The listing builds one solid part. Answer for the finished solid, in the listing's coordinates (mm). Face numbers are marked on the shaded views. A direction names the side the tool comes from. Coordinates: 2 decimals unless noted, no trailing zeros. Write each loop counter-clockwise with the first axis right and the second up, starting at its lowest first coordinate (ties: lowest second). Pieces come first, ordered by that corner, then holes.
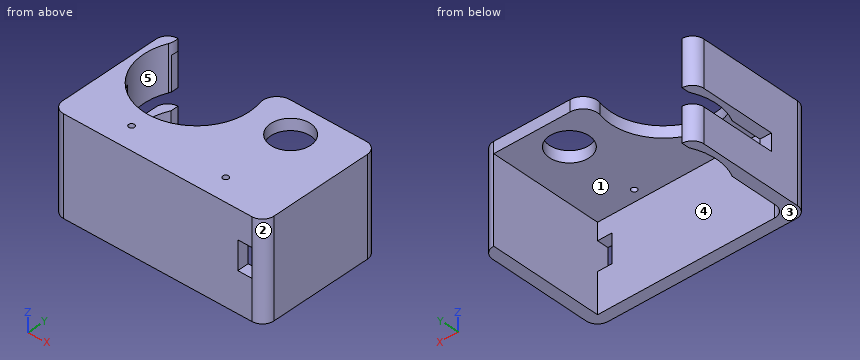
from build123d import *

# Parameters (mm, degrees)
ESQUISSE2_W             = 74
ESQUISSE2_H             = 44
BOSS_EXTRU_1_DEPTH      = 4
ESQUISSE4_R             = 7
ESQUISSE4_R_2           = 18.5
ESQUISSE4_R_3           = 1
ENL_V_MAT_EXTRU_1_DEPTH = 71.394310982
BOSS_EXTRU_2_START      = -4
BOSS_EXTRU_2_DEPTH      = 34
CONG_1_R                = 4
ESQUISSE7_W             = 6
ESQUISSE7_H             = 30
ENL_V_MAT_EXTRU_2_DEPTH = 10
CONG_2_START            = -13
CONG_2_DEPTH            = 18
ESQUISSE8_W             = 5
ESQUISSE8_H             = 10
ENL_V_MAT_EXTRU_3_DEPTH = 77.369560077


with BuildPart() as part:
    # Esquisse2 → Boss.-Extru.1 (new body)
    with BuildSketch(Plane.XY):
        with Locations((-20.726161369, 18.08801956)):
            Rectangle(ESQUISSE2_W, ESQUISSE2_H)
    extrude(amount=BOSS_EXTRU_1_DEPTH)

    # Esquisse4 → Enlèv. mat.-Extru.1 (cut, through all)
    with BuildSketch(Plane.XY.offset(4)):
        with Locations((-4.226161369, 29.08801956)):
            Circle(ESQUISSE4_R)
        with Locations((-37.226161369, 29.08801956)):
            Circle(ESQUISSE4_R_2)
        with Locations((-4.226161369, 4.08801956)):
            Circle(ESQUISSE4_R_3)
        with Locations((-37.226161369, 4.08801956)):
            Circle(ESQUISSE4_R_3)
    extrude(amount=-ENL_V_MAT_EXTRU_1_DEPTH, mode=Mode.SUBTRACT)

    # Boss.-Extru.2: read off the stored shape, not the designer's step
    # Boss.-Extru.2 outline → Boss.-Extru.2 (add)
    with BuildSketch(Plane(origin=(0, 0, 0), x_dir=(-1, 0, 0), z_dir=(0, 0, -1)).offset(BOSS_EXTRU_2_START)):
        with BuildLine():
            Line((-12.273838631, 40.08801956), (-16.273838631, 40.08801956))
            Line((-16.273838631, 40.08801956), (-16.273838631, -3.91198044))
            Line((-16.273838631, -3.91198044), (57.726161369, -3.91198044))
            Line((57.726161369, -3.91198044), (57.726161369, 40.08801956))
            Line((57.726161369, 40.08801956), (53.726161369, 40.08801956))
            Line((53.726161369, 40.08801956), (53.726161369, 37.454619825))
            ThreePointArc((53.726161369, 37.454619825), (55.726161369, 29.08801956), (53.726161369, 20.721419295))
            Line((53.726161369, 20.721419295), (53.726161369, 0.08801956))
            Line((53.726161369, 0.08801956), (-12.273838631, 0.08801956))
            Line((-12.273838631, 0.08801956), (-12.273838631, 40.08801956))
        make_face()
    extrude(amount=BOSS_EXTRU_2_DEPTH)

    # Congé1
    cong_1_edges = [part.edges().sort_by_distance(p)[0] for p in [
        (-53.726161369, 0.08801956, -15),
        (-57.726161369, 40.08801956, -15),
        (16.273838631, 40.08801956, -15),
        (16.273838631, -3.91198044, -15),
        (-57.726161369, -3.91198044, -15),
    ]]
    fillet(cong_1_edges, radius=CONG_1_R - 0.0001)  # a hair under: the kernel refuses the full size

    # Esquisse7 → Enlèv. mat.-Extru.2 (cut)
    with BuildSketch(Plane.ZY.offset(57.726161369)):
        with Locations((-15, 25.08801956)):
            Rectangle(ESQUISSE7_W, ESQUISSE7_H)
    extrude(amount=-ENL_V_MAT_EXTRU_2_DEPTH, mode=Mode.SUBTRACT)

    # Congé2: read off the stored shape, not the designer's step
    # Congé2 outline → Congé2 (cut)
    with BuildSketch(Plane.XY.offset(CONG_2_START)):
        with BuildLine():
            Line((-52.10063615, 40.08801956), (-53.726161369, 40.08801956))
            ThreePointArc((-53.726161369, 40.08801956), (-53.604311661, 38.421947689), (-54.038082686, 36.808725593))
            ThreePointArc((-54.038082686, 36.808725593), (-53.153978754, 38.498366704), (-52.10063615, 40.08801956))
        make_face()
        with BuildLine():
            ThreePointArc((-22.351686589, 40.08801956), (-20.5475812, 37.09270341), (-19.339309991, 33.811423815))
            ThreePointArc((-19.339309991, 33.811423815), (-18.466274294, 38.139004751), (-14.505025834, 40.08801956))
            Line((-14.505025834, 40.08801956), (-22.351686589, 40.08801956))
        make_face()
    extrude(amount=CONG_2_DEPTH, mode=Mode.SUBTRACT)

    # Esquisse8 → Enlèv. mat.-Extru.3 (cut, through all)
    with BuildSketch(Plane(origin=(0, 0.08801956, 0), x_dir=(1, 0, 0), z_dir=(0, 1, 0))):
        with Locations((9.773838631, 11)):
            Rectangle(ESQUISSE8_W, ESQUISSE8_H)
    extrude(amount=-ENL_V_MAT_EXTRU_3_DEPTH, mode=Mode.SUBTRACT)


solid = part.part
1. Flat-ended cylindrical pins translate along their axes: P1, Ø1, axis at x = -1, z = -13, coming from the +Y side; P2, Ø12.5, axis at x = -4.23, y = 29.09, coming from the -Z side; P3, Ø1.3, axis at y = 39, z = -22, coming from the +X side; P4, Ø2.5, axis at y = 39, z = -5, coming from the +X side. Find the tip coordinate at first contact, or state that the pin passes through.
Results found:
P1: stops at y = 0.09
P2: passes through
P3: stops at x = 15.57
P4: stops at x = 15.91
2. Section B-B on y = 18 is taken. Give the vertices of the cut face in (x, z), then the cut area to 3 significant figures.
Results found:
outline: (-57.73, -30) - (-53.73, -30) - (-53.73, -18) - (-57.73, -18) - close; (-57.73, -12) - (-53.73, -12) - (-53.73, 0) - (-52.04, 0) - (-52.04, 4) - (-57.73, 4) - close; (-22.42, 0) - (12.27, 0) - (12.27, -30) - (16.27, -30) - (16.27, 4) - (-22.42, 4) - close
area: 394 mm2
3. A tool of negligible diameter and unlimited length cuts with its end or side. For the marked faces 1 and 2, from which of +Z, -Z, +X, -X, +Y, -Y can it reach the whole face along a straight path? Write none if from no direction.
Results found:
face 1: -Z, +Y
face 2: +Z, -Z, +X, -Y
4. Find the intervals of material crossed by L1, parallel to X at y = 14, z = -5; L2, parallel to X at y = 28.5, z = -8; L3, parallel to Y at x = 9, z = -1.5, in increasing order.
Results found:
L1: x = -57.73 to -53.73, 12.27 to 16.27
L2: x = -57.73 to -55.72, 12.27 to 16.27
L3: y = -3.91 to 0.09
5. For a pull along Y with two mould halves and no side action, classify the marked faces 3, 4 and 5 as pulls with the +Y half, pulls with the -Y half, needs draft (parallel to the pull), parting line crosses it, or undercut.
Results found:
face 3: needs draft
face 4: pulls with the +Y half
face 5: undercut
6. Section D-D on x = 0 is taken. Give the vertices of the cut face in (y, z), then the cut area to 3 significant figures.
Results found:
outline: (-3.91, -30) - (0.09, -30) - (0.09, 0) - (23.51, 0) - (23.51, 4) - (-3.91, 4) - close; (34.67, 0) - (40.09, 0) - (40.09, 4) - (34.67, 4) - close
area: 251 mm2
